For this review, take the finished solid that the model builds, in its own axes (mm). A direction names the side the tool comes from. Round coordinates to 2 decimals unless told otherwise and drop trailing zeros. Order: outer loops, then holes, each group sorted by start corner. A loop starts at its lowest first (then second) coordinate and runs counter-clockwise, first axis right, second up. Notation, with made-up numbers: (-35, 80) -> (-8, 80) arc R24 ccw to (-8, 99) -> close; hole circle Ø4 at (32.25, 56). An arc over 180 degrees is marked (long way). Answer in a Markdown table with one row per item.
```python
from build123d import *

# Parameters (mm, degrees)
SKETCH1_R           = 1.5748
BOSS_EXTRUDE1_DEPTH = 0.381


with BuildPart() as part:
    # Sketch1 → Boss-Extrude1 (new body)
    with BuildSketch(Plane.XY):
        with BuildLine():
            Line((1.9812, 2.927177815), (1.9812, 7.866528823))
            ThreePointArc((1.9812, 7.866528823), (2.063659626, 8.053851807), (2.257498427, 8.119548151))
            Line((2.257498427, 8.119548151), (8.340740358, 7.583436046))
            ThreePointArc((8.340740358, 7.583436046), (8.465877984, 7.653948909), (8.445206773, 7.796090354))
            ThreePointArc((8.445206773, 7.796090354), (0, 11.4935), (-8.445206773, 7.796090354))
            ThreePointArc((-8.445206773, 7.796090354), (-8.465877984, 7.653948909), (-8.340740358, 7.583436046))
            Line((-8.340740358, 7.583436046), (-2.257498427, 8.119548151))
            ThreePointArc((-2.257498427, 8.119548151), (-2.063659626, 8.053851806), (-1.9812, 7.866528823))
            Line((-1.9812, 7.866528823), (-1.9812, 2.927177815))
            ThreePointArc((-1.9812, 2.927177815), (-2.007526398, 2.814569063), (-2.081048276, 2.725303483))
            ThreePointArc((-2.081048276, 2.725303483), (-2.96960111, 1.7145), (-3.400706187, 0.439588932))
            ThreePointArc((-3.400706187, 0.439588932), (-3.441251508, 0.331284328), (-3.525610349, 0.252180623))
            Line((-3.525610349, 0.252180623), (-7.8032138, -2.217494881))
            ThreePointArc((-7.8032138, -2.217494881), (-8.006670076, -2.239744242), (-8.160484179, -2.104723089))
            Line((-8.160484179, -2.104723089), (-10.737818442, 3.431575013))
            ThreePointArc((-10.737818442, 3.431575013), (-10.861453187, 3.504690945), (-10.974215684, 3.415718428))
            ThreePointArc((-10.974215684, 3.415718428), (-9.953662978, -5.74675), (-2.529008911, -11.211808783))
            ThreePointArc((-2.529008911, -11.211808783), (-2.395575203, -11.158639854), (-2.397078085, -11.015011059))
            Line((-2.397078085, -11.015011059), (-5.902985752, -6.014825062))
            ThreePointArc((-5.902985752, -6.014825062), (-5.94301045, -5.814107564), (-5.8220138, -5.649033941))
            Line((-5.8220138, -5.649033941), (-1.544410349, -3.179358437))
            ThreePointArc((-1.544410349, -3.179358437), (-1.43372511, -3.145853391), (-1.319657911, -3.164892415))
            ThreePointArc((-1.319657911, -3.164892415), (0, -3.429), (1.319657911, -3.164892415))
            ThreePointArc((1.319657911, -3.164892415), (1.43372511, -3.145853391), (1.544410349, -3.179358437))
            Line((1.544410349, -3.179358437), (5.8220138, -5.649033941))
            ThreePointArc((5.8220138, -5.649033941), (5.94301045, -5.814107564), (5.902985752, -6.014825062))
            Line((5.902985752, -6.014825062), (2.397078085, -11.015011059))
            ThreePointArc((2.397078085, -11.015011059), (2.395575203, -11.158639854), (2.529008911, -11.211808783))
            ThreePointArc((2.529008911, -11.211808783), (9.953662978, -5.74675), (10.974215684, 3.415718428))
            ThreePointArc((10.974215684, 3.415718428), (10.861453187, 3.504690945), (10.737818442, 3.431575013))
            Line((10.737818442, 3.431575013), (8.160484179, -2.104723089))
            ThreePointArc((8.160484179, -2.104723089), (8.006670076, -2.239744242), (7.8032138, -2.217494881))
            Line((7.8032138, -2.217494881), (3.525610349, 0.252180623))
            ThreePointArc((3.525610349, 0.252180623), (3.441251508, 0.331284328), (3.400706187, 0.439588932))
            ThreePointArc((3.400706187, 0.439588932), (2.96960111, 1.7145), (2.081048276, 2.725303483))
            ThreePointArc((2.081048276, 2.725303483), (2.007526398, 2.814569063), (1.9812, 2.927177815))
        make_face()
        Circle(SKETCH1_R, mode=Mode.SUBTRACT)
    extrude(amount=BOSS_EXTRUDE1_DEPTH)


solid = part.part
```
Q1. Take a section at A-A, the plane x = 4.25. Write out the cut boundary in (y, z), then the cut area to 3 significant figures.
Answer key:
| item | result |
|---|---|
| outline | (-10.68, 0) -> (-8.37, 0) -> (-8.37, 0.38) -> (-10.68, 0.38) -> close; (-4.74, 0) -> (-0.17, 0) -> (-0.17, 0.38) -> (-4.74, 0.38) -> close; (7.94, 0) -> (10.68, 0) -> (10.68, 0.38) -> (7.94, 0.38) -> close |
| area | 3.66 mm^2 |
Q2. The part is to be moulded in two halves that separate along X. For faces 3 (the face through (2.98, 1.7, 0.19)), 4 (the face through (0, -2, 0)), 5 (the face through (0.133, 11.493, 0.188)), 6 (the face through (-2.96, 1.73, 0.19)), say which applies: +X half, -X half, draft (parallel to the pull), parting line (faces both ways), or undercut.
Answer key:
| item | result |
|---|---|
| face 3 | undercut |
| face 4 | draft |
| face 5 | parting line |
| face 6 | undercut |
Q3. To check wall thickness, follow probe 1 along Y at (x, z) = (-4.75, 0.3); probe 2 along X at (y, z) = (0.5, 0.3); probe 3 along X at (y, z) = (5.75, 0.15). State the ranges of each line that lie inside material, in increasing order.
Answer key:
| item | result |
|---|---|
| probe 1 | y = -10.47 to -7.66, -5.03 to -0.45, 7.9 to 10.47 |
| probe 2 | x = -11.48 to -9.37, -3.39 to -1.49, 1.49 to 3.39, 9.37 to 11.48 |
| probe 3 | x = -1.98 to 1.98 |
Q4. Clearance check with a flat-ended pin moving along its axis: pin 1 Ø1.5 at (x, y) = (-5, 6) entering from -Z. State where the tip first meets the part, or that it passes through.
Answer key:
| item | result |
|---|---|
| pin 1 | passes through |
Q5. Take a section at B-B, the plane x = 8.75. Write out the cut boundary in (y, z).
Answer key:
| item | result |
|---|---|
| outline | (-7.45, 0) -> (-0.84, 0) -> (-0.84, 0.38) -> (-7.45, 0.38) -> close |
Q6. Tool access review of faces 1 (the face through (4.175, -8.48, 0.188)), 2 (the face through (0, -2, 0.381)): name each direction out of +Z, -Z, +X, -X, +Y, -Y from which nothing blocks a thin tool from reaching the whole face with its end or side.
Answer key:
| item | result |
|---|---|
| face 1 | +Z, -Z |
| face 2 | +Z, +X, -X, +Y, -Y |
